from build123d import *

# Parameters (mm, degrees)
ESKIZ_KONTUR_W        = 41.2
ESKIZ_KONTUR_H        = 20.2
PLASTINA_DEPTH        = 5
OTVERSTIYA_DEPTH      = 122.659652126
OTVERSTIYA_DEPTH_BACK = 122.659652126
ESKIZ_OTVERSTIYA_R    = 1.65
ESKIZ_OTVERSTIYA_R_2  = 2.15


with BuildPart() as part:
    # Eskiz_kontur → Plastina (new body)
    with BuildSketch(Plane.XY):
        with BuildLine():
            Line((78.04349, 17.26807), (114.2094, 15.99634))
            ThreePointArc((114.2094, 15.99634), (118.316039529, 14.167943464), (119.999997488, 9.999993404))
            Line((119.999997488, 9.999993404), (119.999997488, -10.000006596))
            ThreePointArc((119.999997488, -10.000006596), (118.31603808, -14.167953985), (114.2094, -15.996349022))
            Line((114.2094, -15.996349022), (78.04349, -17.268079022))
            ThreePointArc((78.04349, -17.268079022), (36.414907375, -12.045919499), (-4.891710116, -19.392564511))
            ThreePointArc((-4.891710116, -19.392564511), (-20.000005367, -4.511e-06), (-4.891710116, 19.392555489))
            ThreePointArc((-4.891710116, 19.392555489), (36.414907375, 12.045910477), (78.04349, 17.26807))
        make_face()
        with Locations((89.85, 0)):
            Rectangle(ESKIZ_KONTUR_W, ESKIZ_KONTUR_H, mode=Mode.SUBTRACT)
    extrude(amount=PLASTINA_DEPTH)

    # Eskiz_otverstiya → Otverstiya (cut, two sides: drawn at the far end of the back side and taken through both)
    with BuildSketch(Plane.XY.offset(-OTVERSTIYA_DEPTH_BACK)):
        with Locations((65.1, -5)):
            Circle(ESKIZ_OTVERSTIYA_R)
        with Locations((114.6, -5)):
            Circle(ESKIZ_OTVERSTIYA_R)
        Circle(ESKIZ_OTVERSTIYA_R_2)
        with Locations((30, 0)):
            Circle(ESKIZ_OTVERSTIYA_R)
        with Locations((52, 0)):
            Circle(ESKIZ_OTVERSTIYA_R)
        with Locations((65.1, 5)):
            Circle(ESKIZ_OTVERSTIYA_R)
        with Locations((114.6, 5)):
            Circle(ESKIZ_OTVERSTIYA_R)
    extrude(amount=OTVERSTIYA_DEPTH + OTVERSTIYA_DEPTH_BACK, mode=Mode.SUBTRACT)


solid = part.part
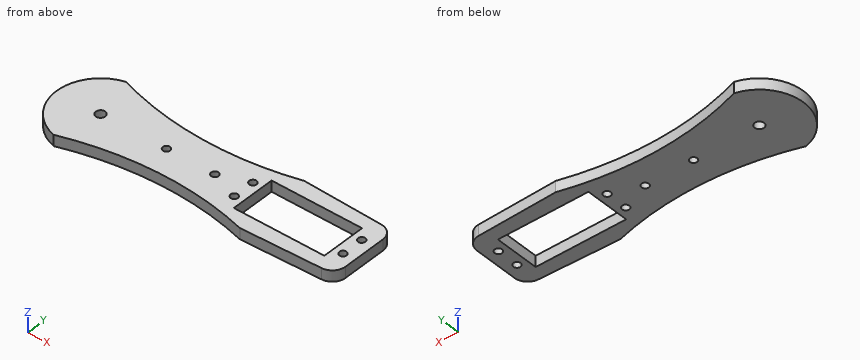
Geometry: final body of the model. Coordinates: model frame, mm. Give positions to 0.01 mm unless a question says otherwise; leave off trailing zeros. Write each loop counter-clockwise with the first axis right and the second up, starting at its lowest first coordinate (ties: lowest second). Pieces come first, ordered by that corner, then holes. Notation, with made-up numbers: (85.5, 23) -> (98.5, 23) arc R10 ccw to (98.5, 32) -> close; hole circle Ø11 at (89.25, 33.5). An arc over 180 degrees is marked (long way). Answer in a Markdown table with one row per item.
(1) Pin query (flat end, axial travel): pin 1 (2 mm diameter, centred on x = 114.6, y = 5, fed in from +Z); pin 2 (2.5 mm diameter, centred on y = 0, z = 1.5, fed in from -X); pin 3 (2 mm diameter, centred on y = -13, z = 2.5, fed in from -X); pin 4 (4 mm diameter, centred on x = 30, y = 0, fed in from +Z). Return the tip coordinate at first contact, or that it passes through.
Answers below:
| item | result |
|---|---|
| pin 1 | through |
| pin 2 | x = -20 |
| pin 3 | x = -16 |
| pin 4 | z = 5 |
(2) Section query D-D on y = 5. Return loops of the section in (x, z), then the cut area to 3 significant figures.
Answers below:
| item | result |
|---|---|
| outline | (-19.36, 0) -> (63.45, 0) -> (63.45, 5) -> (-19.36, 5) -> close; (66.75, 0) -> (69.25, 0) -> (69.25, 5) -> (66.75, 5) -> close; (110.45, 0) -> (112.95, 0) -> (112.95, 5) -> (110.45, 5) -> close; (116.25, 0) -> (120, 0) -> (120, 5) -> (116.25, 5) -> close |
| area | 458 mm^2 |
(3) Section query B-B on y = -14. Return loops of the section in (x, z).
Answers below:
| item | result |
|---|---|
| outline | (-14.28, 0) -> (16.42, 0) -> (16.42, 5) -> (-14.28, 5) -> close; (63.58, 0) -> (118.47, 0) -> (118.47, 5) -> (63.58, 5) -> close |
(4) Ray query, line 1 along X through (y, z) = (0, 1.8); line 2 along X through (y, z) = (-5, 3.95); line 3 along Y through (x, z) = (114.6, 1.15). Return the intervals inside material, ascending. Write a range as [from, to].
Answers below:
| item | result |
|---|---|
| line 1 | [-20, -2.15], [2.15, 28.35], [31.65, 50.35], [53.65, 69.25], [110.45, 120] |
| line 2 | [-19.36, 63.45], [66.75, 69.25], [110.45, 112.95], [116.25, 120] |
| line 3 | [-15.97, -6.65], [-3.35, 3.35], [6.65, 15.97] |
(5) Section query C-C on x = 0. Return loops of the section in (y, z).
Answers below:
| item | result |
|---|---|
| outline | (-17.84, 0) -> (-2.15, 0) -> (-2.15, 5) -> (-17.84, 5) -> close; (2.15, 0) -> (17.84, 0) -> (17.84, 5) -> (2.15, 5) -> close |
(6) Section query A-A on z = 2.55. State how many separate pieces and enclosed holes the cut face has, then the cut area to 3 significant figures.
Answers below:
| item | result |
|---|---|
| separate pieces | 1 |
| enclosed holes | 8 |
| area | 3,250 mm^2 |
